Check sheet for the modelled part. Datum: model origin and axes. Units: mm. Face numbers are marked on the shaded views. A direction names the side the tool comes from. Round coordinates to 2 decimals unless told otherwise and drop trailing zeros. Loops run counter-clockwise (first coordinate to the right, second up) from the corner with the lowest first, then second, coordinate; pieces in that order, holes last. Notation, with made-up numbers: M 50,-7 L 62,-7 A15 cw 62,-3 Z; hole C 74,63 d10. An arc over 180 degrees is marked long. One line per question, with ' | ' between items. Start each with the question number.
(1) Go/stop test with flat-tipped pins: P1, Ø14, axis at x = 1, y = -48, coming from the +Z side; P2, Ø6.5, axis at x = -39, y = -13, coming from the +Z side; P3, Ø5, axis at x = -7, y = -68, coming from the +Z side. Record where each tip stops, or that it passes through.
(2) Thickness scan on probe 1 along Y at (x, z) = (-3.5, -39); probe 2 along Y at (x, z) = (23.5, 19); probe 3 along Z at (x, y) = (0, -47). Record the ranges inside material, lowest first. Write a range as [from, to].
(3) Section check B-B (x = 0). Record the boundary of the cut face in (y, z).
(4) Section check A-A (z = -12). Record the boundary of the cut face in (x, y), and give its area (3 significant figures).
(5) Section check D-D (z = 40). Record the boundary of the cut face in (x, y).
(6) Tool access check on the marked faces 5 and 6. Record the directions out of +Z, -Z, +X, -X, +Y, -Y that give a thin tool (end or side, any length) a straight path to the whole face; none if there is none.
(7) Section check C-C (z = 0). Record the boundary of the cut face in (x, y), and give its area (3 significant figures).
(8) Draft check along X on the marked faces 1, 2, 3 and 4. Enter one of: +X half, -X half, draft (parallel to the pull), parting line (faces both ways), or undercut.
```python
from build123d import *

# Parameters (mm, degrees)
F0_W      = 101.603322
F0_H      = 101.60333
F1_DEPTH  = 101.6
F2_T      = -6.35
F3_W      = 12.7
F3_H      = 12.7
F4_DEPTH  = 38.1
F5_W      = 12.7
F5_H      = 12.7
F6_DEPTH  = 38.1
F7_W      = 12.7
F7_H      = 12.7
F8_DEPTH  = 38.1
F9_W      = 12.7
F9_H      = 12.7
F10_DEPTH = 38.1
F11_W     = 12.7
F11_H     = 12.7
F12_DEPTH = 50.8
F13_R     = 3.310042
F14_DEPTH = 25.4


with BuildPart() as f1:
    # F0 (on Front) → F1 (new body)
    with BuildSketch(Plane.XZ):
        Rectangle(F0_W, F0_H)
    extrude(amount=F1_DEPTH)

    # F2
    f2_openings = [f1.faces().sort_by_distance(p)[0] for p in [
        (0, -50.8, 50.801665),
    ]]
    offset(amount=F2_T, openings=f2_openings)

    # F3 (on face) → F4 (join)
    with BuildSketch(Plane.XY.offset(-44.451665)):
        with Locations((-38.101661, -12.7)):
            Rectangle(F3_W, F3_H)
    extrude(amount=F4_DEPTH)

    # F5 (on face) → F6 (join)
    with BuildSketch(Plane.XY.offset(-44.451665)):
        with Locations((38.101661, -12.7)):
            Rectangle(F5_W, F5_H)
    extrude(amount=F6_DEPTH)

    # F7 (on face) → F8 (join)
    with BuildSketch(Plane.XY.offset(-44.451665)):
        with Locations((-38.101661, -88.9)):
            Rectangle(F7_W, F7_H)
    extrude(amount=F8_DEPTH)

    # F9 (on face) → F10 (join)
    with BuildSketch(Plane.XY.offset(-44.451665)):
        with Locations((38.101661, -88.9)):
            Rectangle(F9_W, F9_H)
    extrude(amount=F10_DEPTH)

    # F11 (on face) → F12 (join)
    with BuildSketch(Plane.XY.offset(-44.451665)):
        with Locations((0, -49.202401)):
            Rectangle(F11_W, F11_H)
    extrude(amount=F12_DEPTH)

    # F13 (on face) → F14 (cut)
    with BuildSketch(Plane.XZ.offset(55.552401)):
        Circle(F13_R)
    extrude(amount=-F14_DEPTH, mode=Mode.SUBTRACT)


solid = f1.part
```
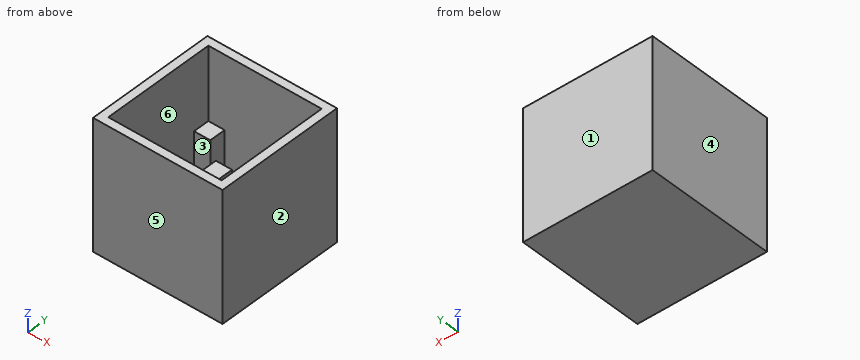
The answers:
1) P1: z = 6.35 | P2: z = -6.35 | P3: z = -44.45
2) probe 1: [-101.6, -95.25], [-55.55, -42.85], [-6.35, 0] | probe 2: [-101.6, -95.25], [-6.35, 0] | probe 3: [-50.8, -3.31], [3.31, 6.35]
3) outline: M -101.6,-50.8 L 0,-50.8 L 0,50.8 L -6.35,50.8 L -6.35,-44.45 L -42.85,-44.45 L -42.85,-3.31 L -55.55,-3.31 L -55.55,-44.45 L -95.25,-44.45 L -95.25,50.8 L -101.6,50.8 Z; M -55.55,3.31 L -42.85,3.31 L -42.85,6.35 L -55.55,6.35 Z
4) outline: M -50.8,-101.6 L 50.8,-101.6 L 50.8,0 L -50.8,0 Z; M -6.35,-55.55 L 6.35,-55.55 L 6.35,-42.85 L -6.35,-42.85 Z; hole M -44.45,-82.55 L -31.75,-82.55 L -31.75,-95.25 L 31.75,-95.25 L 31.75,-82.55 L 44.45,-82.55 L 44.45,-19.05 L 31.75,-19.05 L 31.75,-6.35 L -31.75,-6.35 L -31.75,-19.05 L -44.45,-19.05 Z | area: 3,230 mm²
5) outline: M -50.8,-101.6 L 50.8,-101.6 L 50.8,0 L -50.8,0 Z; hole M -44.45,-95.25 L 44.45,-95.25 L 44.45,-6.35 L -44.45,-6.35 Z
6) face 5: +Z, -Z, +X, -X, -Y | face 6: +Z
7) outline: M -50.8,-101.6 L 50.8,-101.6 L 50.8,0 L -50.8,0 Z; M -6.35,-55.55 L -3.31,-55.55 L -3.31,-42.85 L -6.35,-42.85 Z; M 3.31,-55.55 L 6.35,-55.55 L 6.35,-42.85 L 3.31,-42.85 Z; hole M -44.45,-95.25 L 44.45,-95.25 L 44.45,-6.35 L -44.45,-6.35 Z | area: 2,500 mm²
8) face 1: draft | face 2: +X half | face 3: undercut | face 4: -X half
